The figure shows three views and two pictorial views of one solid part (mm, origin at its lowest corner). Answer the questions. A direction names the side the tool comes from. Coordinates: 2 decimals unless noted, no trailing zeros. Loops run counter-clockwise (first coordinate to the right, second up) from the corner with the lowest first, then second, coordinate; pieces in that order, holes last. Notation, with made-up numbers: M -25.75,12 L 13.25,12 A22 ccw 13.25,35 Z; hole C 89.5,86 d1. An arc over 180 degrees is marked long. Answer as a JSON object with one key per item and string values. Group by question number.
1. A cutting plane is placed at B-B on z = 75. Give the vertices of the cut face in (x, y), and give its area (3 significant figures).
2. Given pin 1 (2 mm diameter, centred on y = 16, z = 63, fed in from +X); pin 2 (1 mm diameter, centred on y = 13, z = 28, fed in from -X); pin 3 (12 mm diameter, centred on x = 109.5, y = 7, fed in from -Z), each flat-ended and moving along its own axis, determine where each tip first touches the part or whether it passes through.
3. A cutting plane is placed at A-A on x = 140. Give the vertices of the cut face in (y, z).
4. A cutting plane is placed at C-C on x = 22.5. Give the vertices of the cut face in (y, z).
5. For the marked faces 1 and 2, determine the directions among +Z, -Z, +X, -X, +Y, -Y from which every point of the face is accessible in a straight line to the end or side of a thin tool.
6. Straight lines are drawn through the part: L1, parallel to X at y = 4.75, z = 75; L2, parallel to X at y = 2.25, z = 65; L3, parallel to Z at x = 22.5, y = 5.25. For each, find the intervals that lie inside material, in ascending order.
7. A cutting plane is placed at D-D on z = 48.5. Give the vertices of the cut face in (x, y), and give its area (3 significant figures).
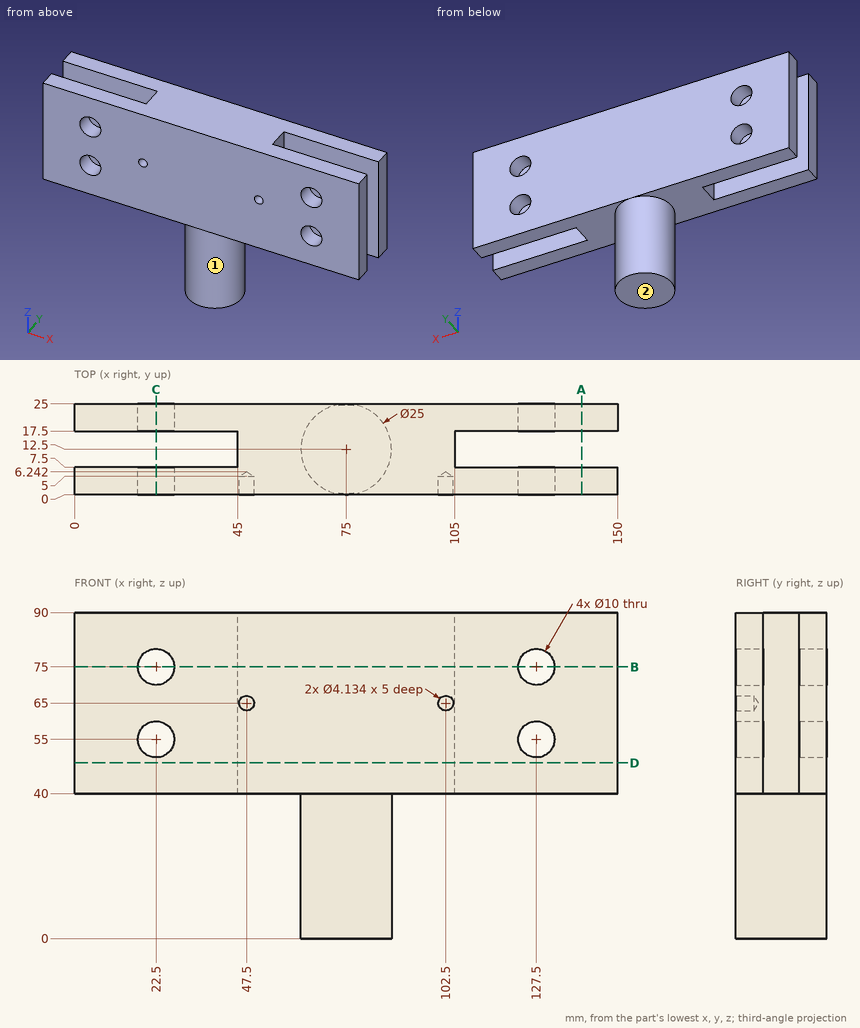
From the geometry:
{
 "1": {"outline": "M 0,0 L 17.5,0 L 17.5,7.5 L 0,7.5 Z; M 0,17.5 L 17.5,17.5 L 17.5,25 L 0,25 Z; M 27.5,0 L 122.5,0 L 122.5,7.5 L 105,7.5 L 105,17.5 L 122.5,17.5 L 122.5,25 L 27.5,25 L 27.5,17.5 L 45,17.5 L 45,7.5 L 27.5,7.5 Z; M 132.5,0 L 150,0 L 150,7.5 L 132.5,7.5 Z; M 132.5,17.5 L 150,17.5 L 150,25 L 132.5,25 Z", "area": "2,550 mm²"},
 "2": {"pin 1": "stops at x = 105", "pin 2": "stops at x = 62.5", "pin 3": "stops at z = 40"},
 "3": {"outline": "M 0,40 L 7.5,40 L 7.5,90 L 0,90 Z; M 17.5,40 L 25,40 L 25,90 L 17.5,90 Z"},
 "4": {"outline": "M 0,40 L 7.5,40 L 7.5,50 L 0,50 Z; M 0,60 L 7.5,60 L 7.5,70 L 0,70 Z; M 0,80 L 7.5,80 L 7.5,90 L 0,90 Z; M 17.5,40 L 25,40 L 25,50 L 17.5,50 Z; M 17.5,60 L 25,60 L 25,70 L 17.5,70 Z; M 17.5,80 L 25,80 L 25,90 L 17.5,90 Z"},
 "5": {"face 1": "-Z", "face 2": "-Z, +X, -X, +Y, -Y"},
 "6": {"L1": "x = 0 to 17.5, 27.5 to 122.5, 132.5 to 150", "L2": "x = 0 to 45.43, 49.57 to 100.43, 104.57 to 150", "L3": "z = 40 to 50, 60 to 70, 80 to 90"},
 "7": {"outline": "M 0,0 L 150,0 L 150,7.5 L 105,7.5 L 105,17.5 L 150,17.5 L 150,25 L 0,25 L 0,17.5 L 45,17.5 L 45,7.5 L 0,7.5 Z", "area": "2,850 mm²"}
}
